Verification items for the finished model (mm, model axes). A direction names the side the tool comes from. Coordinates: 2 decimals unless noted, no trailing zeros. Loops run counter-clockwise (first coordinate to the right, second up) from the corner with the lowest first, then second, coordinate; pieces in that order, holes last. Notation, with made-up numbers: (82.5, 70) - (140.5, 70) arc R32 ccw to (140.5, 98) - close; hole circle Ø10 at (-29.75, -5.75). An arc over 180 degrees is marked (long way). One line per item, written item: value. Start each with the question number.
(1) Section check A-A (x = 116.5). Record the boundary of the cut face in (y, z).
(2) Section check D-D (x = 32.5). Record the boundary of the cut face in (y, z), plus the area to 3 significant figures.
(3) Thickness scan on probe 1 along Y at (x, z) = (38, 0.5); probe 2 along Y at (x, z) = (29, 1); probe 3 along X at (y, z) = (48, 0.75). Record the ranges inside material, lowest first. Write a range as [from, to].
(4) Draft check along X on faces 1 (the face through (216.368, 70.448, 5.07)), 2 (the face through (84, 36, 0)), 3 (the face through (172.82, 52.57, 5.07)). Enter one of: +X half, -X half, draft (parallel to the pull), parting line (faces both ways), or undercut.
(5) Section check B-B (x = 10). Record the boundary of the cut face in (y, z).
(6) Set-up check for faces 4 (the face through (68.46, 33.61, 5.07)), 5 (the face through (0, 41, 5)): record each of +Z, -Z, +X, -X, +Y, -Y from which the full face is reachable in a straight line by a thin tool's end or side.
(7) Section check C-C (z = 8). Count the separate pieces of the cut face and the enclosed holes in it, plus the area to 3 significant figures.
(8) Gauge pin test, flat ends, axial feed: P1, Ø5.5, axis at x = 195, y = 50.54, coming from the -Z side; P2, Ø3, axis at x = 69.5, z = 7.5, coming from the -Y side; P3, Ø3, axis at y = 15.5, z = 7, coming from the +X side; P4, Ø6, axis at x = 63, z = 7.5, coming from the +Y side. Record the tip position at first contact, or that the pin passes through.
```python
from build123d import *

# Parameters (mm, degrees)
ESQUISSE1_W                             = 220
ESQUISSE1_H                             = 90
BOSS_EXTRU_1_DEPTH                      = 10
ESQUISSE2_OUTSIDE_W                     = 269.582
ESQUISSE2_OUTSIDE_H                     = 139.582
ENL_V_MAT_EXTRU_1_DEPTH                 = 238.907545067
ENL_V_MAT_EXTRU_2_DEPTH                 = 238.907545067
CONG_1_R                                = 15
ESQUISSE4_R                             = 3.305
ENL_V_MAT_EXTRU_3_DEPTH                 = 238.90731446
PER_AGE_POUR_CROUS_AUTO_BLOQUANTS_300_D = 4.7625
PER_AGE_POUR_CROUS_AUTO_BLOQUANTS_3_2_D = 4.7625
ENL_V_MAT_EXTRU_4_DEPTH                 = 10
CONG_2_R                                = 10


with BuildPart() as part:
    # Esquisse1 → Boss.-Extru.1 (new body)
    with BuildSketch(Plane.XY):
        with Locations((110, 45)):
            Rectangle(ESQUISSE1_W, ESQUISSE1_H)
    extrude(amount=BOSS_EXTRU_1_DEPTH)

    # Esquisse2 outside → Enlèv. mat.-Extru.1 (cut, through all)
    with BuildSketch(Plane.XY.offset(10)):
        with Locations((110, 45)):
            Rectangle(ESQUISSE2_OUTSIDE_W, ESQUISSE2_OUTSIDE_H)
        Polygon((220, 73.248936833), (125, 90), (45, 83.000906918), (0, 66.622246376), (0, 16.622246376), (28.790575259, 0), (113.790575259, 0), (135.121280108, 9.946671025), (150.121280108, 35.927433138), (220, 48.248936833), align=None, mode=Mode.SUBTRACT)
    extrude(amount=-ENL_V_MAT_EXTRU_1_DEPTH, mode=Mode.SUBTRACT)

    # Esquisse3 → Enlèv. mat.-Extru.2 (cut, through all)
    with BuildSketch(Plane.XY.offset(10)):
        Polygon((124.495639968, 21.542522439), (141.732730573, 51.398039143), (122.912069568, 74.760032194), (61.263110797, 69.366447183), (106.536954459, 13.168249856), align=None)
        Polygon((96.247958869, 10), (73.776753989, 37.893395035), (62.988565413, 29.202319765), align=None)
        Polygon((20, 25.154266119), (20, 36.701271503), (40, 36.701271503), (86.247958869, 10), (28.660254038, 20.154266119), align=None)
        Polygon((20, 54.021779578), (49.998184356, 36.702319765), (65, 48.78793618), (48.421740656, 69.366447183), (20, 59.021779578), align=None)
    extrude(amount=-ENL_V_MAT_EXTRU_2_DEPTH, mode=Mode.SUBTRACT)

    # Congé1
    # the kernel refuses this fillet: 15 mm, written as the material it takes off along each edge
    with BuildSketch(Plane(origin=(220, 73.248936833, 41.466236169), x_dir=(-0.9848077530122094, 0.17364817766692334, 0), z_dir=(0, 0, -1))) as cong_1_piece_1:
        with BuildLine():
            CenterArc((CONG_1_R * 0.839099631177, -CONG_1_R), CONG_1_R, 90, 80)
            Line((-CONG_1_R * 0.145708121835, -CONG_1_R * 0.826351822333), (0, 0))
            Line((0, 0), (CONG_1_R * 0.839099631177, 0))
        make_face()
    extrude(amount=72.932472338, mode=Mode.SUBTRACT)
    with BuildSketch(Plane(origin=(220, 48.248936833, 41.466236169), x_dir=(-0.9848077530122079, -0.17364817766693147, 0), z_dir=(0, 0, -1))) as cong_1_piece_2:
        with BuildLine():
            CenterArc((CONG_1_R * 0.839099631177, CONG_1_R), CONG_1_R, 190, 80)
            Line((-CONG_1_R * 0.145708121835, CONG_1_R * 0.826351822333), (0, 0))
            Line((0, 0), (CONG_1_R * 0.839099631177, 0))
        make_face()
    extrude(amount=72.932472338, mode=Mode.SUBTRACT)

    # Esquisse4 → Enlèv. mat.-Extru.3 (cut, through all)
    with BuildSketch(Plane.XY.offset(10)):
        with Locations((194.999750621, 50.537155323)):
            Circle(ESQUISSE4_R)
        with Locations((169.766644599, 53.836955846)):
            Circle(ESQUISSE4_R)
    extrude(amount=-ENL_V_MAT_EXTRU_3_DEPTH, mode=Mode.SUBTRACT)

    # Per_age pour _crous auto-bloquants 300 (through all)
    with Locations(Plane.XY.offset(10)):
        with Locations((102.584612496, 80.510258923)):
            Hole(PER_AGE_POUR_CROUS_AUTO_BLOQUANTS_300_D / 2)

    # Per_age pour _crous auto-bloquants 3 2 (through all)
    with Locations(Plane.XY.offset(10)):
        with Locations((10, 56.521779578), (10, 26.722713174)):
            Hole(PER_AGE_POUR_CROUS_AUTO_BLOQUANTS_3_2_D / 2)

    # Esquisse10 → Enlèv. mat.-Extru.4 (cut)
    with BuildSketch(Plane.XY.offset(10)):
        Polygon((146.450960741, 78.662842867), (145.356977222, 72.458554023), (165.348574608, 68.933496016), (166.442558127, 75.13778486), align=None)
    extrude(amount=-ENL_V_MAT_EXTRU_4_DEPTH, mode=Mode.SUBTRACT)

    # Congé2
    cong_2_edges = [part.edges().sort_by_distance(p)[0] for p in [
        (150.121280108, 35.927433138, 5),
    ]]
    fillet(cong_2_edges, radius=CONG_2_R)


solid = part.part
```
Responses:
1. outline: (1.26, 0) - (17.81, 0) - (17.81, 10) - (1.26, 10) - close; (74.2, 0) - (89.26, 0) - (89.26, 10) - (74.2, 10) - close
2. outline: (0, 0) - (19.48, 0) - (19.48, 10) - (0, 10) - close; (36.7, 0) - (46.8, 0) - (46.8, 10) - (36.7, 10) - close; (63.57, 0) - (78.45, 0) - (78.45, 10) - (63.57, 10) - close
2. area: 445 mm²
3. probe 1: y = [0, 18.51], [36.7, 43.63], [65.57, 80.45]
3. probe 2: y = [0, 20.09], [36.7, 48.83], [62.3, 77.18]
3. probe 3: x = [0, 30.43], [64.02, 78.48], [139.77, 192.88], [197.12, 212.76]
4. face 1: +X half
4. face 2: draft
4. face 3: undercut
5. outline: (10.85, 0) - (24.34, 0) - (24.34, 10) - (10.85, 10) - close; (29.1, 0) - (54.14, 0) - (54.14, 10) - (29.1, 10) - close; (58.9, 0) - (70.26, 0) - (70.26, 10) - (58.9, 10) - close
6. face 4: +Z, -Z
6. face 5: +Z, -Z, -X, +Y, -Y
7. separate pieces: 1
7. enclosed holes: 10
7. area: 9,480 mm²
8. P1: passes through
8. P2: stops at y = 0
8. P3: stops at x = 139.19
8. P4: stops at y = 84.84
